Model file for the job. Use its own axes, mm. Face numbers are marked on the shaded views. A direction names the side the tool comes from. Round coordinates to 2 decimals unless told otherwise and drop trailing zeros. Order: outer loops, then holes, each group sorted by start corner. A loop starts at its lowest first (then second) coordinate and runs counter-clockwise, first axis right, second up. Notation, with made-up numbers: (34, 89) -> (88, 89) arc R25 cw to (88, 119) -> close; hole circle Ø6 at (-21, 12.25). An arc over 180 degrees is marked (long way). Answer as CSV lines item,"result".
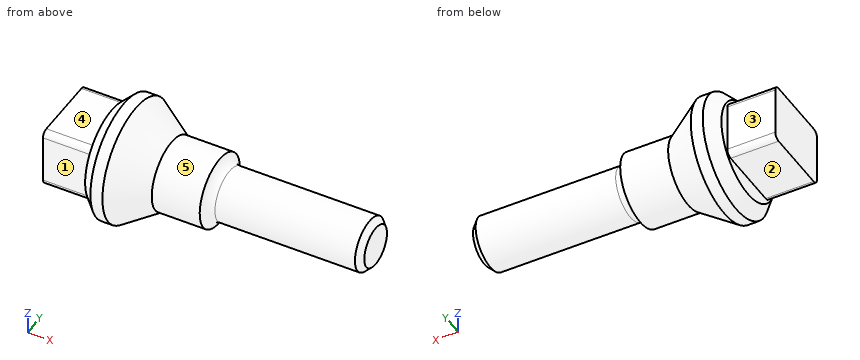
```python
from build123d import *

# Parameters (mm, degrees)
SKETCH1_W           = 10
SKETCH1_H           = 50
SKETCH1_W_2         = 40
SKETCH1_H_2         = 30
SKETCH1_W_3         = 121.767034814
SKETCH1_H_3         = 22
SKETCH2_W           = 50
SKETCH2_H           = 62.449979984
BOSS_EXTRUDE1_DEPTH = 40
FILLET2_R           = 5
FILLET3_R           = 5
CHAMFER1_SIZE       = 5


with BuildPart() as part:
    # Sketch1 → Revolve1 (revolve)
    with BuildSketch(Plane.XY, mode=Mode.PRIVATE) as revolve1_sk:
        Polygon((10, 0), (0, 0), (0, -40), (10, -50), align=None)
        with Locations((15, -25)):
            Rectangle(SKETCH1_W, SKETCH1_H)
        Polygon((50, 0), (20, 0), (20, -50), (50, -30), align=None)
        with Locations((70, -15)):
            Rectangle(SKETCH1_W_2, SKETCH1_H_2)
        with BuildLine():
            Line((98.232965186, 0), (90, 0))
            Line((90, 0), (90, -30))
            ThreePointArc((90, -30), (92.493154306, -24.329399341), (98.232965186, -22))
            Line((98.232965186, -22), (98.232965186, 0))
        make_face()
        with Locations((159.116482593, -11)):
            Rectangle(SKETCH1_W_3, SKETCH1_H_3)
    revolve(revolve1_sk.sketch.rotate(Axis((0, 0, 0), (1, 0, 0)), 270), axis=Axis((0, 0, 0), (1, 0, 0)))

    # Sketch2 → Boss-Extrude1 (add)
    with BuildSketch(Plane.ZY):
        Rectangle(SKETCH2_W, SKETCH2_H)
    extrude(amount=BOSS_EXTRUDE1_DEPTH)

    # Fillet2
    fillet2_edges = [part.edges().sort_by_distance(p)[0] for p in [
        (-20, 31.224989992, 25),
    ]]
    fillet(fillet2_edges, radius=FILLET2_R)

    # Fillet3
    fillet3_edges = [part.edges().sort_by_distance(p)[0] for p in [
        (-20, -31.224989992, 25),
        (-20, 31.224989992, -25),
        (-20, -31.224989992, -25),
    ]]
    fillet(fillet3_edges, radius=FILLET3_R)

    # Chamfer1
    chamfer1_edges = [part.edges().sort_by_distance(p)[0] for p in [
        (220, 0, -22),
    ]]
    chamfer(chamfer1_edges, length=CHAMFER1_SIZE)


solid = part.part
```
Q1. Tool access for the marked faces 1, 2, 3, 4 and 5: list every direction of +Z, -Z, +X, -X, +Y, -Y with a clear straight run to the whole face (end or side of a thin tool).
Checks:
face 1,"+Z, -Z, -X, -Y"
face 2,"-Z, -X, +Y, -Y"
face 3,"+Z, -Z, -X, +Y"
face 4,"+Z, -X, +Y, -Y"
face 5,"+X"
Q2. Saw through at D-D (x = 58.5). Write the cut outline in (y, z).
Checks:
outline,"circle Ø60 at (0, 0)"
Q3. Saw through at B-B (y = 0). Write the cut outline in (x, z), plus the area to 3 significant figures.
Checks:
outline,"(-40, -25) -> (0, -25) -> (0, -40) -> (10, -50) -> (20, -50) -> (50, -30) -> (90, -30) arc R8.24 cw to (98.23, -22) -> (215, -22) -> (220, -17) -> (220, 17) -> (215, 22) -> (98.23, 22) arc R8.24 cw to (90, 30) -> (50, 30) -> (20, 50) -> (10, 50) -> (0, 40) -> (0, 25) -> (-40, 25) -> close"
area,"14,400 mm²"
Q4. Saw through at C-C (x = 149). Write the cut outline in (y, z).
Checks:
outline,"circle Ø44 at (0, 0)"
Q5. Wall check: L1, parallel to Z at x = -0.5, y = -8; L2, parallel to Z at x = 99, y = -1; L3, parallel to Y at x = -25, z = -4. Give the ranges that are in metal, low to high. Write a range as [from, to].
Checks:
L1,"[-25, 25]"
L2,"[-21.98, 21.98]"
L3,"[-31.22, 31.22]"
Q6. Flat gauge pins, fed straight in: pin 1 (20 mm diameter, centred on x = -23.5, z = 1.5, fed in from +Y) (3 decimals); pin 2 (2 mm diameter, centred on x = 41.5, z = -16.5, fed in from +Y); pin 3 (12 mm diameter, centred on x = 77.5, z = 33, fed in from -Y). Where does each tip first touch, or does it go through?
Checks:
pin 1,"y = 31.225"
pin 2,"y = 32.52"
pin 3,"y = -13.08"
Q7. Saw through at A-A (z = 0). Write the cut outline in (x, y).
Checks:
outline,"(-40, -31.22) -> (0, -31.22) -> (0, -40) -> (10, -50) -> (20, -50) -> (50, -30) -> (90, -30) arc R8.24 cw to (98.23, -22) -> (215, -22) -> (220, -17) -> (220, 17) -> (215, 22) -> (98.23, 22) arc R8.24 cw to (90, 30) -> (50, 30) -> (20, 50) -> (10, 50) -> (0, 40) -> (0, 31.22) -> (-40, 31.22) -> close"
